Can you work these out from the drawing? Everything is in mm from the part's minimum corner. A direction names the side the tool comes from. Give positions to 0.01 mm unless a question says otherwise; leave off trailing zeros. Order: outer loops, then holes, each group sorted by start corner. A loop starts at its lowest first (then second) coordinate and runs counter-clockwise, first axis right, second up. Notation, with made-up numbers: (34, -18.75) - (82, -18.75) arc R17 ccw to (82, 14.25) - close; hole circle Ø10 at (-5, -32.75). An arc over 180 degrees is marked (long way). Answer as a JSON object with one key per item and string values.
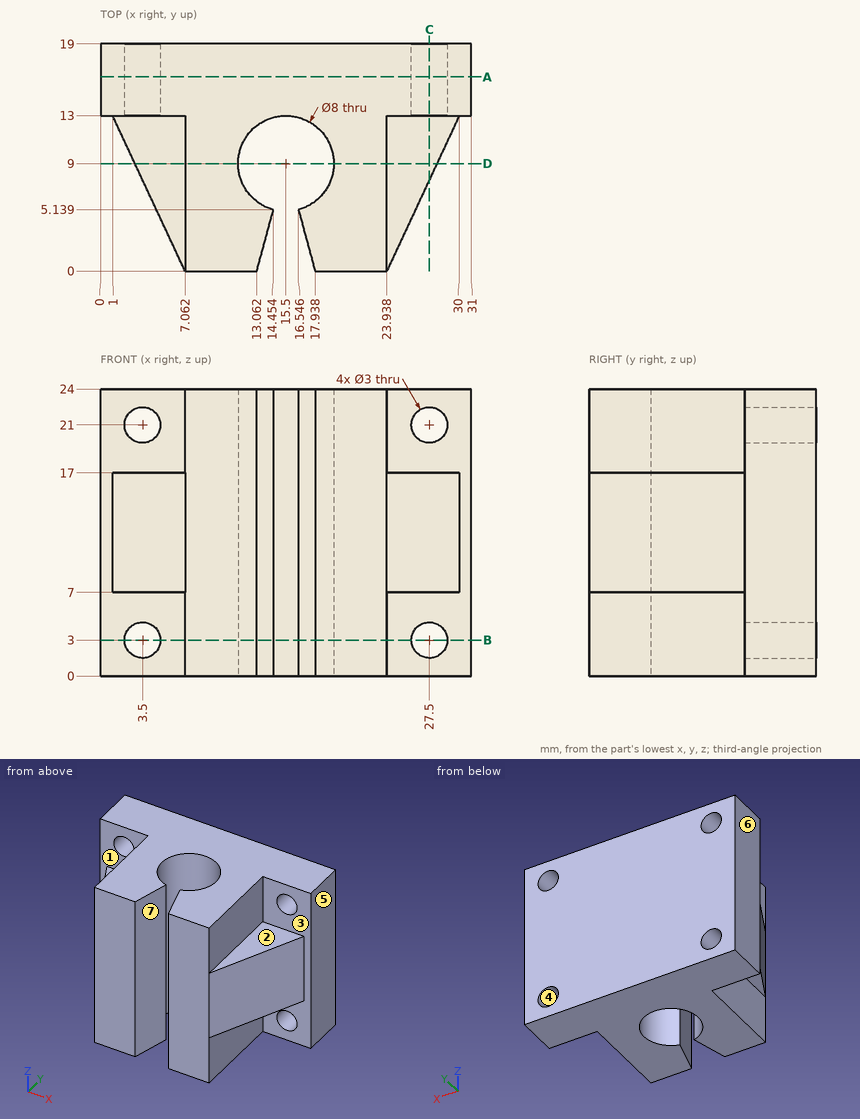
Q1. We'd pull the mould along X, two halves only. Please class the marked faces 4, 5, 6 and 7: released by +X, released by -X, zero draft, split by the parting line, or undercut.
Recorded:
{"face 4": "undercut", "face 5": "released by +X", "face 6": "released by -X", "face 7": "undercut"}
Q2. If we section it at C-C, the plane x = 27.5: Please give me the cut outline in (y, z).
Recorded:
{"outline": "(7.64, 7) - (13, 7) - (13, 4.5) - (19, 4.5) - (19, 19.5) - (13, 19.5) - (13, 17) - (7.64, 17) - close; (13, 0) - (19, 0) - (19, 1.5) - (13, 1.5) - close; (13, 22.5) - (19, 22.5) - (19, 24) - (13, 24) - close"}
Q3. Which directions (+Z, -Z, +X, -X, +Y, -Y) give clear straight access to the entire face, cutting with the end or side of a thin tool? Please do the marked faces 1, 2 and 3.
Recorded:
{"face 1": "-X, -Y", "face 2": "+Z, +X, -Y", "face 3": "+X, -Y"}
Q4. If we section it at D-D, the plane y = 9: Please give me the cut outline in (x, z) (1 decimal).
Recorded:
{"outline": "(2.9, 7) - (7.1, 7) - (7.1, 0) - (11.5, 0) - (11.5, 24) - (7.1, 24) - (7.1, 17) - (2.9, 17) - close; (19.5, 0) - (23.9, 0) - (23.9, 7) - (28.1, 7) - (28.1, 17) - (23.9, 17) - (23.9, 24) - (19.5, 24) - close"}
Q5. I'm going to push flat-ended pins straight in: pin 1 Ø1.8 at (x, y) = (26.5, 9) entering from +Z; pin 2 Ø2 at (y, z) = (4.5, 4.5) entering from -X; pin 3 Ø5.5 at (y, z) = (9.5, 21) entering from +X. Where does each tip first touch, or does it pass through?
Recorded:
{"pin 1": "stops at z = 17", "pin 2": "stops at x = 7.06", "pin 3": "stops at x = 23.94"}
Q6. I need wall thicknesses on L1, parallel to Z at x = 27.5, y = 14.25; L2, parallel to X at y = 9, z = 5; L3, parallel to X at y = 15.5, z = 4.25. Which ranges of each line are inside material? Lowest first, please.
Recorded:
{"L1": "z = 0 to 1.5, 4.5 to 19.5, 22.5 to 24", "L2": "x = 7.06 to 11.5, 19.5 to 23.94", "L3": "x = 0 to 2.67, 4.33 to 26.67, 28.33 to 31"}
Q7. If we section it at A-A, the plane y = 16.25: Please give me the cut outline in (x, z), then the cut area to 3 significant figures.
Recorded:
{"outline": "(0, 0) - (31, 0) - (31, 24) - (0, 24) - close; hole circle Ø3 at (3.5, 3); hole circle Ø3 at (3.5, 21); hole circle Ø3 at (27.5, 3); hole circle Ø3 at (27.5, 21)", "area": "716 mm^2"}
Q8. If we section it at B-B, the plane z = 3: Please give me the cut outline in (x, y).
Recorded:
{"outline": "(0, 13) - (2, 13) - (2, 19) - (0, 19) - close; (5, 13) - (7.06, 13) - (7.06, 0) - (13.06, 0) - (14.45, 5.14) arc R4 cw (long way) to (16.55, 5.14) - (17.94, 0) - (23.94, 0) - (23.94, 13) - (26, 13) - (26, 19) - (5, 19) - close; (29, 13) - (31, 13) - (31, 19) - (29, 19) - close"}
